Build history of the part. All positions in model axes, mm. Round coordinates to 2 decimals unless told otherwise and drop trailing zeros. Write each loop counter-clockwise with the first axis right and the second up, starting at its lowest first coordinate (ties: lowest second). Pieces come first, ordered by that corner, then holes. Notation, with made-up numbers: (-13.75, -6.5) -> (38.25, -6.5) arc R14 ccw to (38.25, 17.5) -> close; hole circle Ø10 at (88, 47.5). An arc over 180 degrees is marked (long way). Return JSON: item names as keys, results as strings.
from build123d import *

# Parameters (mm, degrees)
SKETCH_1_R      = 1.45
SKETCH_1_R_2    = 60
EXTRUDE_1_DEPTH = 3
FILLET_2_R      = 3


with BuildPart() as part:
    # 草图1 → 凸台-拉伸1 (new body)
    with BuildSketch(Plane(origin=(0, 0, 0), x_dir=(1, 0, 0), z_dir=(0, 1, 0))):
        with BuildLine():
            Line((-30, -67.372564891), (-30, -92.5))
            Line((-30, -92.5), (30, -92.5))
            Line((30, -92.5), (30, -67.372564891))
            ThreePointArc((30, -67.372564891), (52.149125113, -52.149125113), (67.372564891, -30))
            Line((67.372564891, -30), (92.5, -30))
            Line((92.5, -30), (92.5, 2.5))
            Line((92.5, 2.5), (112.5, 12.5))
            Line((112.5, 12.5), (112.5, 27.5))
            Line((112.5, 27.5), (92.5, 37.5))
            Line((92.5, 37.5), (63.504428979, 37.5))
            ThreePointArc((63.504428979, 37.5), (-4.219374226, 73.629201959), (-67.372564891, 30))
            Line((-67.372564891, 30), (-92.5, 30))
            Line((-92.5, 30), (-92.5, -30))
            Line((-92.5, -30), (-67.372564891, -30))
            ThreePointArc((-67.372564891, -30), (-52.149125113, -52.149125113), (-30, -67.372564891))
        make_face()
        with Locations(Location((-20, -85, 0), (0, 0, 270))):
            Circle(SKETCH_1_R, mode=Mode.SUBTRACT)
        with Locations(Location((0, -85, 0), (0, 0, 270))):
            Circle(SKETCH_1_R, mode=Mode.SUBTRACT)
        with Locations(Location((0, -63.75, 0), (0, 0, 270))):
            Circle(SKETCH_1_R, mode=Mode.SUBTRACT)
        with Locations(Location((-45.078057301, -45.078057301, 0), (0, 0, 270))):
            Circle(SKETCH_1_R, mode=Mode.SUBTRACT)
        with Locations(Location((-85, -20, 0), (0, 0, 270))):
            Circle(SKETCH_1_R, mode=Mode.SUBTRACT)
        with Locations(Location((20, -85, 0), (0, 0, 270))):
            Circle(SKETCH_1_R, mode=Mode.SUBTRACT)
        with Locations(Location((45.078057301, -45.078057301, 0), (0, 0, 270))):
            Circle(SKETCH_1_R, mode=Mode.SUBTRACT)
        with Locations(Location((85, -20, 0), (0, 0, 270))):
            Circle(SKETCH_1_R, mode=Mode.SUBTRACT)
        with Locations(Location((-85, 0, 0), (0, 0, 270))):
            Circle(SKETCH_1_R, mode=Mode.SUBTRACT)
        with Locations(Location((-63.75, 0, 0), (0, 0, 270))):
            Circle(SKETCH_1_R, mode=Mode.SUBTRACT)
        with Locations(Location((-85, 20, 0), (0, 0, 270))):
            Circle(SKETCH_1_R, mode=Mode.SUBTRACT)
        with Locations(Location((0, 0, 0), (0, 0, 270))):
            Circle(SKETCH_1_R_2, mode=Mode.SUBTRACT)
        with Locations(Location((-45.078057301, 45.078057301, 0), (0, 0, 270))):
            Circle(SKETCH_1_R, mode=Mode.SUBTRACT)
        with Locations(Location((0, 63.75, 0), (0, 0, 270))):
            Circle(SKETCH_1_R, mode=Mode.SUBTRACT)
        with Locations(Location((63.75, 0, 0), (0, 0, 270))):
            Circle(SKETCH_1_R, mode=Mode.SUBTRACT)
        with Locations(Location((85, 7.5, 0), (0, 0, 270))):
            Circle(SKETCH_1_R, mode=Mode.SUBTRACT)
        with Locations(Location((45.078057301, 45.078057301, 0), (0, 0, 270))):
            Circle(SKETCH_1_R, mode=Mode.SUBTRACT)
        with Locations(Location((85, 32.5, 0), (0, 0, 270))):
            Circle(SKETCH_1_R, mode=Mode.SUBTRACT)
        with Locations(Location((97.5, 20, 0), (0, 0, 270))):
            Circle(SKETCH_1_R, mode=Mode.SUBTRACT)
        with Locations(Location((107.5, 20, 0), (0, 0, 270))):
            Circle(SKETCH_1_R, mode=Mode.SUBTRACT)
    extrude(amount=EXTRUDE_1_DEPTH)

    # 圆角2
    fillet_2_edges = [part.edges().sort_by_distance(p)[0] for p in [
        (63.504428979, 1.5, -37.5),
        (92.5, 1.5, -37.5),
        (112.5, 1.5, -27.5),
        (112.5, 1.5, -12.5),
        (92.5, 1.5, -2.5),
        (92.5, 1.5, 30),
        (67.372564891, 1.5, 30),
        (30, 1.5, 67.372564891),
        (30, 1.5, 92.5),
        (-30, 1.5, 92.5),
        (-30, 1.5, 67.372564891),
        (-67.372564891, 1.5, 30),
        (-92.5, 1.5, 30),
        (-92.5, 1.5, -30),
        (-67.372564891, 1.5, -30),
    ]]
    fillet(fillet_2_edges, radius=FILLET_2_R)


solid = part.part
Q1. Pin check, flat tip, straight feed: pin 1 Ø0.9 at (x, y) = (82, 1) entering from +Z. Stop position of the tip, or through.
Verdict:
{"pin 1": "stops at z = 30"}
Q2. Saw through at B-B on z = 35. List the corners of the cut face in (x, y).
Verdict:
{"outline": "(-64.92, 0) -> (-48.73, 0) -> (-48.73, 3) -> (-64.92, 3) -> close; (48.73, 0) -> (64.92, 0) -> (64.92, 3) -> (48.73, 3) -> close"}
Q3. Two-plate mould, pull along X, no slides. Class faces 1 (the cylindrical face through (51.9, 1.479, 52.397)), 2 (the cylindrical face through (2.64, 1.48, -59.94)), 3 (the flat face through (40, 3, 46)): +X half, -X half, draft (parallel to the pull), parting line (faces both ways), or undercut.
Verdict:
{"face 1": "+X half", "face 2": "undercut", "face 3": "draft"}
Q4. Wall check: L1, parallel to X at y = 1.7, z = 85; L2, parallel to X at y = 2.2, z = 0. Give the ranges that are in metal, low to high.
Verdict:
{"L1": "x = -30 to -21.45, -18.55 to -1.45, 1.45 to 18.55, 21.45 to 30", "L2": "x = -92.5 to -86.45, -83.55 to -65.2, -62.3 to -60, 60 to 62.3, 65.2 to 92.5"}
Q5. Saw through at D-D on x = -80. List the corners of the cut face in (y, z), then the cut area to 3 significant figures.
Verdict:
{"outline": "(0, -30) -> (3, -30) -> (3, 30) -> (0, 30) -> close", "area": "180 mm²"}
Q6. Saw through at A-A on z = 4. List the corners of the cut face in (x, y).
Verdict:
{"outline": "(-92.5, 0) -> (-59.87, 0) -> (-59.87, 3) -> (-92.5, 3) -> close; (59.87, 0) -> (92.5, 0) -> (92.5, 3) -> (59.87, 3) -> close"}
Q7. Saw through at C-C on y = 2. Count the separate pieces of the cut face and the enclosed holes in it, then the cut area to 3 significant figures.
Verdict:
{"separate pieces": "1", "enclosed holes": "20", "area": "10,100 mm²"}
